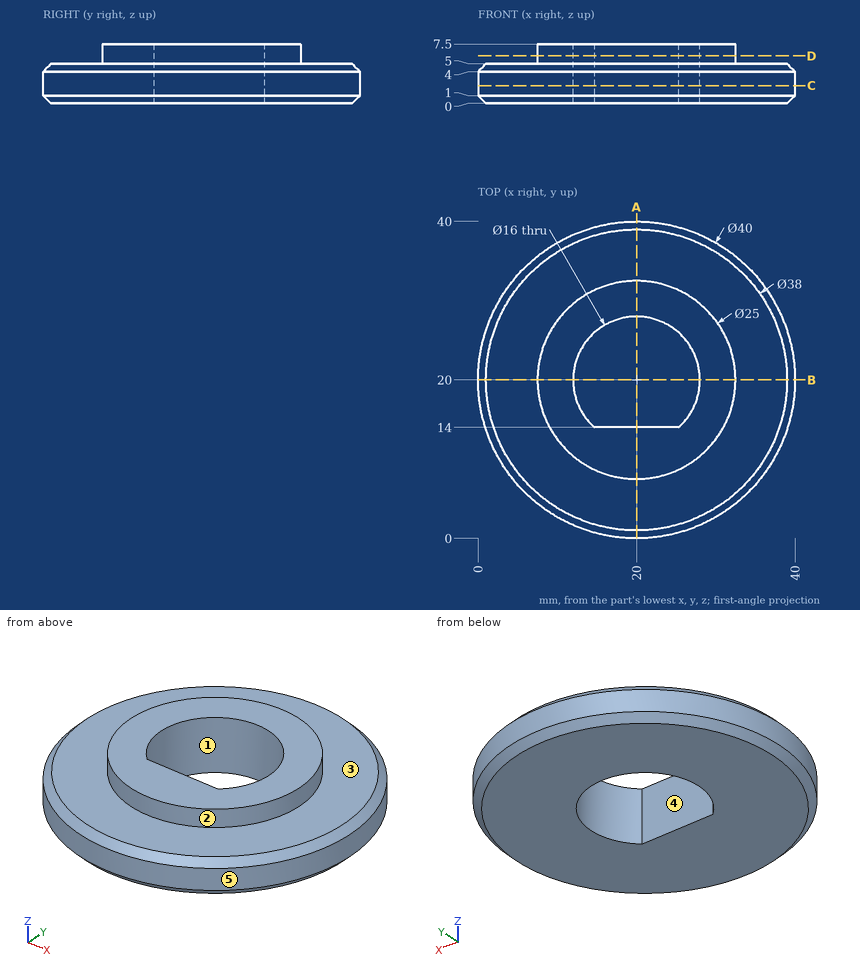
Could you check a few things on this drawing? It's one solid part, dimensions in mm from its lowest x, y, z. A direction names the side the tool comes from. Give positions to 0.01 mm unless a question says otherwise; leave off trailing zeros. Order: outer loops, then holes, each group sorted by start corner. A loop starts at its lowest first (then second) coordinate and runs counter-clockwise, first axis right, second up.
1. Suppose I cut it at B-B (y = 20). Write out the boundary of the cut face in (x, z), plus the area to 4 significant figures.
Answers below:
outline: (0, 1) - (1, 0) - (12, 0) - (12, 7.5) - (7.5, 7.5) - (7.5, 5) - (1, 5) - (0, 4) - close; (28, 0) - (39, 0) - (40, 1) - (40, 4) - (39, 5) - (32.5, 5) - (32.5, 7.5) - (28, 7.5) - close
area: 140.5 mm2
2. I need wall thicknesses on L1, parallel to Y at x = 20, z = 2.75; L2, parallel to Z at x = 13, y = 31; L3, parallel to X at y = 16, z = 3.75. Which ranges of each line are inside material? Lowest first, please.
Answers below:
L1: y = 0 to 14, 28 to 40
L2: z = 0 to 5
L3: x = 0.4 to 13.07, 26.93 to 39.6
3. Suppose I cut it at D-D (z = 6). Write out the boundary of the cut face in (x, y).
Answers below:
outline: circle Ø25 at (20, 20); hole (14.71, 14) - (25.29, 14) arc R8 ccw (long way) to start
4. Suppose I cut it at A-A (x = 20). Write out the boundary of the cut face in (y, z).
Answers below:
outline: (0, 1) - (1, 0) - (14, 0) - (14, 7.5) - (7.5, 7.5) - (7.5, 5) - (1, 5) - (0, 4) - close; (28, 0) - (39, 0) - (40, 1) - (40, 4) - (39, 5) - (32.5, 5) - (32.5, 7.5) - (28, 7.5) - close
5. Thinking about a two-plate mould opening in X: for the marked faces 3, 4 and 5, which applies, +X half, -X half, draft (parallel to the pull), parting line (faces both ways), or undercut?
Answers below:
face 3: draft
face 4: undercut
face 5: parting line
6. For pin 1 (2 mm diameter, centred on x = 28.5, z = 3.5, fed in from +Y); pin 2 (1 mm diameter, centred on y = 18.5, z = 3, fed in from +X) (3 decimals); pin 3 (1 mm diameter, centred on x = 4.5, y = 20.5, fed in from +Z), each with a flat end and sliding along its axis, tell me the tip position at first contact or that it passes through.
Answers below:
pin 1: stops at y = 38.54
pin 2: stops at x = 39.975
pin 3: stops at z = 5
7. Which directions (+Z, -Z, +X, -X, +Y, -Y) give clear straight access to the entire face, cutting with the end or side of a thin tool? Please do the marked faces 1 and 2.
Answers below:
face 1: +Z, -Z
face 2: +Z
8. Suppose I cut it at C-C (z = 2.25). Write out the boundary of the cut face in (x, y), plus the area to 3 significant figures.
Answers below:
outline: circle Ø40 at (20, 20); hole (14.71, 14) - (25.29, 14) arc R8 ccw (long way) to start
area: 1,070 mm2
